Geometry: final body of the model. Coordinates: model frame, mm. A direction names the side the tool comes from. Give positions to 0.01 mm unless a question says otherwise; leave off trailing zeros. Loops run counter-clockwise (first coordinate to the right, second up) from the corner with the lowest first, then second, coordinate; pieces in that order, holes last. Notation, with made-up numbers: (86, 43.25) - (91, 43.25) arc R18 ccw to (91, 53.25) - close; hole circle Ø10 at (40, 23.5). An arc over 180 degrees is marked (long way). Use CSV: the item, a comma, the result in double quotes. Start each with the question number.
```python
from build123d import *

# Parameters (mm, degrees)
SKETCH1_W           = 36.5
SKETCH1_H           = 22.6
BOSS_EXTRUDE2_DEPTH = 10
SHELL2_T            = -1
SKETCH2_R           = 8.4
CUT_EXTRUDE1_DEPTH  = 10
SKETCH3_W           = 3
SKETCH3_H           = 10
CUT_EXTRUDE3_DEPTH  = 10
SKETCH4_W           = 15
SKETCH4_H           = 6
BOSS_EXTRUDE3_DEPTH = 9
SKETCH5_R           = 1.75
CUT_EXTRUDE4_DEPTH  = 18


with BuildPart() as part:
    # Sketch1 → Boss-Extrude2 (new body)
    with BuildSketch(Plane.XY):
        Rectangle(SKETCH1_W, SKETCH1_H)
    extrude(amount=BOSS_EXTRUDE2_DEPTH)

    # Shell2
    shell2_openings = [part.faces().sort_by_distance(p)[0] for p in [
        (0, 0, 0),
    ]]
    offset(amount=SHELL2_T, openings=shell2_openings, kind=Kind.INTERSECTION)

    # Sketch2 → Cut-Extrude1 (cut)
    with BuildSketch(Plane(origin=(0, 0, 9), x_dir=(-1, 0, 0), z_dir=(0, 0, -1))):
        with Locations((4.75, 0)):
            Circle(SKETCH2_R)
    extrude(amount=-CUT_EXTRUDE1_DEPTH, mode=Mode.SUBTRACT)

    # Sketch3 → Cut-Extrude3 (cut)
    with BuildSketch(Plane(origin=(18.25, 0, 0), x_dir=(0, 0, -1), z_dir=(1, 0, 0))):
        with Locations((-3.4, 0)):
            Rectangle(SKETCH3_W, SKETCH3_H)
    extrude(amount=-CUT_EXTRUDE3_DEPTH, mode=Mode.SUBTRACT)

    # Sketch4 → Boss-Extrude3 (add)
    with BuildSketch(Plane(origin=(0, 0, 9), x_dir=(-1, 0, 0), z_dir=(0, 0, -1))):
        with Locations((7.5, 14.3)):
            Rectangle(SKETCH4_W, SKETCH4_H)
        with Locations((7.5, -14.3)):
            Rectangle(SKETCH4_W, SKETCH4_H)
    extrude(amount=BOSS_EXTRUDE3_DEPTH)

    # Sketch5 → Cut-Extrude4 (cut)
    with BuildSketch(Plane(origin=(0, 0, 0), x_dir=(-1, 0, 0), z_dir=(0, 0, -1))):
        with Locations((7.455294422, 14.124015169)):
            Circle(SKETCH5_R)
        with Locations((7.455294422, -14.296167592)):
            Circle(SKETCH5_R)
    extrude(amount=-CUT_EXTRUDE4_DEPTH, mode=Mode.SUBTRACT)


solid = part.part
```
Item 1: Section D-D (y = -13). Output: boundary loops of the cut face in (x, z), plus the area to 3 significant figures.
Item 2: Ray query, probe 1 along Y at (x, z) = (9, 4.5); probe 2 along X at (y, z) = (-9.5, 5.25); probe 3 along Y at (x, z) = (-4.75, 9.4). Return the intervals inside material, ascending.
Item 3: Section B-B (x = -4.75). Output: boundary loops of the cut face in (y, z).
Item 4: Section C-C (x = 6). Output: boundary loops of the cut face in (y, z).
Item 5: Section A-A (y = 0). Output: boundary loops of the cut face in (x, z), plus the area to 3 significant figures.
Item 6: Mould query, pull axis X, two halves, no side actions, for faces 6 (the flat face through (-15, 14, 5)), 7 (the flat face through (-7, -12, 9)), 8 (the flat face through (17.25, -0.1, 5.4)). Classes: pulls with the +X half, pulls with the -X half, needs draft (parallel to the pull), parting line crosses it, or undercut.
Item 7: Reachability of faces 1 (the flat face through (4, 2, 9)), 2 (the flat face through (-5.7, 15, 9)), 3 (the flat face through (0, 14, 5)), 4 (the flat face through (18, 0, 4.9)), 5 (the flat face through (-15, -14, 5)) from +Z, -Z, +X, -X, +Y, -Y: full face, straight path, thin tool, end or side. Return the list, or none.
Item 8: Pin query (flat end, axial travel): pin 1 Ø3 at (x, y) = (-5, 15.5) entering from +Z; pin 2 Ø1.8 at (y, z) = (-14, 6) entering from -X; pin 3 Ø3 at (y, z) = (14.5, 5) entering from +X; pin 4 Ø13.5 at (x, y) = (-4.75, 0) entering from +Z. Return the tip coordinate at first contact, or that it passes through.
Outcome:
1,outline,"(-15, 0) - (-8.63, 0) - (-8.63, 9) - (-15, 9) - close; (-6.28, 0) - (0, 0) - (0, 9) - (-6.28, 9) - close"
1,area,"114 mm2"
2,probe 1,"y = -11.3 to -10.3, 10.3 to 11.3"
2,probe 2,"x = -18.25 to -17.25, 17.25 to 18.25"
2,probe 3,"y = -11.3 to -8.4, 8.4 to 11.3"
3,outline,"(-17.3, 0) - (-10.3, 0) - (-10.3, 9) - (-8.4, 9) - (-8.4, 10) - (-11.3, 10) - (-11.3, 9) - (-17.3, 9) - close; (8.4, 9) - (10.3, 9) - (10.3, 0) - (17.3, 0) - (17.3, 9) - (11.3, 9) - (11.3, 10) - (8.4, 10) - close"
4,outline,"(-11.3, 0) - (-10.3, 0) - (-10.3, 9) - (10.3, 9) - (10.3, 0) - (11.3, 0) - (11.3, 10) - (-11.3, 10) - close"
5,outline,"(-18.25, 0) - (-17.25, 0) - (-17.25, 9) - (-13.15, 9) - (-13.15, 10) - (-18.25, 10) - close; (3.65, 9) - (17.25, 9) - (17.25, 4.9) - (18.25, 4.9) - (18.25, 10) - (3.65, 10) - close; (17.25, 0) - (18.25, 0) - (18.25, 1.9) - (17.25, 1.9) - close"
5,area,"34.7 mm2"
6,face 6,"pulls with the -X half"
6,face 7,"needs draft"
6,face 8,"undercut"
7,face 1,"-Z"
7,face 2,"+Z, +X, -X, +Y"
7,face 3,"+Z, -Z, +X, +Y"
7,face 4,"+X"
7,face 5,"+Z, -Z, -X, -Y"
8,pin 1,"stops at z = 9"
8,pin 2,"stops at x = -15"
8,pin 3,"stops at x = 0"
8,pin 4,"passes through"
